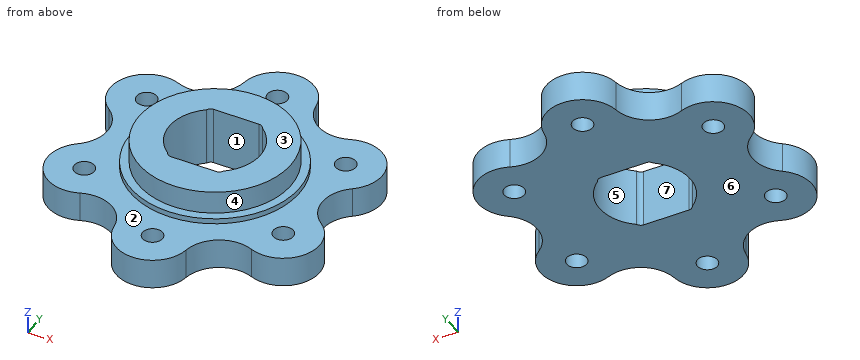
```python
from build123d import *

# Parameters (mm, degrees)
EXTRUDE_1_DEPTH     = 5
SKETCH_1_3_R        = 13.883
EXTRUDE_2_DEPTH     = 5.9
SKETCH_1_4_R        = 12.5
EXTRUDE_3_DEPTH     = 9.7
CUT_EXTRUDE_1_DEPTH = 35.975617108
M4X0_7_1_D          = 3.3
SKETCH_5_R          = 0.92977942
CUT_EXTRUDE_2_DEPTH = 35.975617108


with BuildPart() as part:
    # ｽｹｯﾁ1 → ﾎﾞｽ - 押し出し1 (new body)
    with BuildSketch(Plane.XY):
        with BuildLine():
            ThreePointArc((5.946480455, 19.799606275), (0, 25), (-5.946480455, 19.799606275))
            ThreePointArc((-5.946480455, 19.799606275), (-8.892960911, 15.403060127), (-14.173721791, 15.049606275))
            ThreePointArc((-14.173721791, 15.049606275), (-21.650635095, 12.5), (-20.120202247, 4.75))
            ThreePointArc((-20.120202247, 4.75), (-17.785921821, 0), (-20.120202247, -4.75))
            ThreePointArc((-20.120202247, -4.75), (-21.650635095, -12.5), (-14.173721791, -15.049606275))
            ThreePointArc((-14.173721791, -15.049606275), (-8.892960911, -15.403060127), (-5.946480455, -19.799606275))
            ThreePointArc((-5.946480455, -19.799606275), (0, -25), (5.946480455, -19.799606275))
            ThreePointArc((5.946480455, -19.799606275), (8.892960911, -15.403060127), (14.173721791, -15.049606275))
            ThreePointArc((14.173721791, -15.049606275), (21.650635095, -12.5), (20.120202247, -4.75))
            ThreePointArc((20.120202247, -4.75), (17.785921821, 0), (20.120202247, 4.75))
            ThreePointArc((20.120202247, 4.75), (21.650635095, 12.5), (14.173721791, 15.049606275))
            ThreePointArc((14.173721791, 15.049606275), (8.892960911, 15.403060127), (5.946480455, 19.799606275))
        make_face()
    extrude(amount=EXTRUDE_1_DEPTH)

    # ｽｹｯﾁ1<3> → ﾎﾞｽ - 押し出し2 (add)
    with BuildSketch(Plane.XY):
        Circle(SKETCH_1_3_R)
    extrude(amount=EXTRUDE_2_DEPTH)

    # ｽｹｯﾁ1<4> → ﾎﾞｽ - 押し出し3 (add)
    with BuildSketch(Plane.XY):
        Circle(SKETCH_1_4_R)
    extrude(amount=EXTRUDE_3_DEPTH)

    # ｽｹｯﾁ1<5> → ｶｯﾄ - 押し出し1 (cut, through all)
    with BuildSketch(Plane.XY):
        with BuildLine():
            Line((-3.741657387, 6.5), (3.741657387, 6.5))
            ThreePointArc((3.741657387, 6.5), (7.5, 0), (3.741657387, -6.5))
            Line((3.741657387, -6.5), (-3.741657387, -6.5))
            ThreePointArc((-3.741657387, -6.5), (-7.5, 0), (-3.741657387, 6.5))
        make_face()
    extrude(amount=CUT_EXTRUDE_1_DEPTH, mode=Mode.SUBTRACT)

    # M4x0.7 ねじ穴1 (through all)
    with Locations(Plane(origin=(0, 19, 0), x_dir=(-1, 0, 0), z_dir=(0, 0, -1))):
        with Locations((0, 0), (-16.454482672, -9.5), (-16.454482672, -28.5), (0, -38), (16.454482672, -28.5), (16.454482672, -9.5)):
            Hole(M4X0_7_1_D / 2)

    # ｽｹｯﾁ5 → ｶｯﾄ - 押し出し2 (cut, through all)
    with BuildSketch(Plane.XY.offset(9.7)):
        with Locations((3.741657387, 5.57022058)):
            Circle(SKETCH_5_R)
        with Locations((3.741657387, -5.57022058)):
            Circle(SKETCH_5_R)
        with Locations((-3.741657387, -5.57022058)):
            Circle(SKETCH_5_R)
        with Locations((-3.741657387, 5.57022058)):
            Circle(SKETCH_5_R)
    extrude(amount=-CUT_EXTRUDE_2_DEPTH, mode=Mode.SUBTRACT)


solid = part.part
```
The listing builds one solid part. Answer for the finished solid, in the listing's coordinates (mm). Face numbers are marked on the shaded views. A direction names the side the tool comes from. Give positions to 0.01 mm unless a question says otherwise; leave off trailing zeros. Order: outer loops, then holes, each group sorted by start corner. A loop starts at its lowest first (then second) coordinate and runs counter-clockwise, first axis right, second up.
Item 1: The part is cut by section A-A, the plane x = 0. Give the vertices of the cut face in (y, z), and give its area (3 significant figures).
From the geometry:
outline: (-25, 0) - (-20.65, 0) - (-20.65, 5) - (-25, 5) - close; (-17.35, 0) - (-6.5, 0) - (-6.5, 9.7) - (-12.5, 9.7) - (-12.5, 5.9) - (-13.88, 5.9) - (-13.88, 5) - (-17.35, 5) - close; (6.5, 0) - (17.35, 0) - (17.35, 5) - (13.88, 5) - (13.88, 5.9) - (12.5, 5.9) - (12.5, 9.7) - (6.5, 9.7) - close; (20.65, 0) - (25, 0) - (25, 5) - (20.65, 5) - close
area: 211 mm2
Item 2: The part is cut by section B-B, the plane y = 0. Give the vertices of the cut face in (x, z), and give its area (3 significant figures).
From the geometry:
outline: (-17.79, 0) - (-7.5, 0) - (-7.5, 9.7) - (-12.5, 9.7) - (-12.5, 5.9) - (-13.88, 5.9) - (-13.88, 5) - (-17.79, 5) - close; (7.5, 0) - (17.79, 0) - (17.79, 5) - (13.88, 5) - (13.88, 5.9) - (12.5, 5.9) - (12.5, 9.7) - (7.5, 9.7) - close
area: 152 mm2
Item 3: Given pin 1 Ø5.5 at (x, y) = (0, 19) entering from +Z; pin 2 Ø5 at (y, z) = (1.5, 3) entering from -X; pin 3 Ø3 at (x, y) = (16.45, 9.5) entering from -Z; pin 4 Ø3 at (x, z) = (3.5, 6) entering from -Y, each flat-ended and moving along its own axis, determine where each tip first touches the part or whether it passes through.
From the geometry:
pin 1: stops at z = 5
pin 2: stops at x = -19.31
pin 3: passes through
pin 4: stops at y = -24.51
Item 4: The part is cut by section D-D, the plane z = 3. Give the vertices of the cut face in (x, y), and give its area (3 significant figures).
From the geometry:
outline: (-20.12, -4.75) arc R6 ccw to (-14.17, -15.05) arc R6 cw to (-5.95, -19.8) arc R6 ccw to (5.95, -19.8) arc R6 cw to (14.17, -15.05) arc R6 ccw to (20.12, -4.75) arc R6 cw to (20.12, 4.75) arc R6 ccw to (14.17, 15.05) arc R6 cw to (5.95, 19.8) arc R6 ccw to (-5.95, 19.8) arc R6 cw to (-14.17, 15.05) arc R6 ccw to (-20.12, 4.75) arc R6 cw to start; hole circle Ø3.3 at (-16.45, -9.5); hole circle Ø3.3 at (-16.45, 9.5); hole (-4.6, -5.92) arc R0.93 ccw to (-3.74, -6.5) - (3.74, -6.5) arc R0.93 ccw to (4.6, -5.92) arc R7.5 ccw to (4.6, 5.92) arc R0.93 ccw to (3.74, 6.5) - (-3.74, 6.5) arc R0.93 ccw to (-4.6, 5.92) arc R7.5 ccw to start; hole circle Ø3.3 at (0, -19); hole circle Ø3.3 at (0, 19); hole circle Ø3.3 at (16.45, -9.5); hole circle Ø3.3 at (16.45, 9.5)
area: 1,250 mm2
Item 5: Find the intervals of material crossed by probe 1 along Y at (x, z) = (0, 8.25); probe 2 along Z at (x, y) = (-20, -13); probe 3 along X at (y, z) = (-3, 3.5), in increasing order.
From the geometry:
probe 1: y = -12.5 to -6.5, 6.5 to 12.5
probe 2: z = 0 to 5
probe 3: x = -18.59 to -6.87, 6.87 to 18.59
Item 6: The part is cut by section C-C, the plane z = 7.75. Give the vertices of the cut face in (x, y).
From the geometry:
outline: circle Ø25 at (0, 0); hole (-4.6, -5.92) arc R0.93 ccw to (-3.74, -6.5) - (3.74, -6.5) arc R0.93 ccw to (4.6, -5.92) arc R7.5 ccw to (4.6, 5.92) arc R0.93 ccw to (3.74, 6.5) - (-3.74, 6.5) arc R0.93 ccw to (-4.6, 5.92) arc R7.5 ccw to start
Item 7: For a pull along X with two mould halves and no side action, classify the marked faces 4, 5, 6 and 7 as pulls with the +X half, pulls with the -X half, needs draft (parallel to the pull), parting line crosses it, or undercut.
From the geometry:
face 4: parting line crosses it
face 5: undercut
face 6: needs draft
face 7: undercut
Item 8: Which of the six approach directions +Z, -Z, +X, -X, +Y, -Y give full straight-line access (tool end or side, diameter ignored) to the marked faces 1, 2 and 3?
From the geometry:
face 1: +Z, -Z
face 2: +Z
face 3: +Z, +X, -X, +Y, -Y
